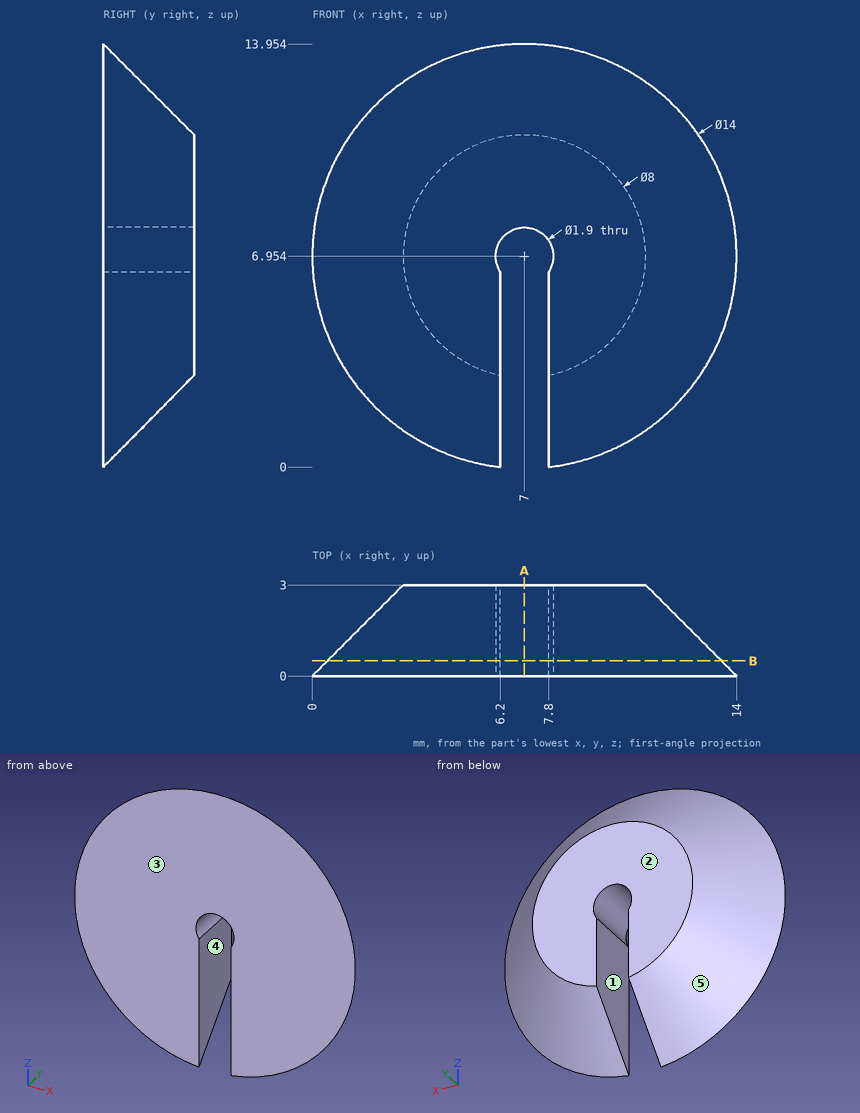
Source: three-view drawing plus pictorial views. Frame: mm from the lowest corner of the part. A direction names the side the tool comes from. Round coordinates to 2 decimals unless told otherwise and drop trailing zeros. Loops run counter-clockwise (first coordinate to the right, second up) from the corner with the lowest first, then second, coordinate; pieces in that order, holes last. Notation, with made-up numbers: M 72.5,14.25 L 111.5,14.25 A20 cw 111.5,36.25 Z; hole C 8,81 d9. An arc over 180 degrees is marked long. Put each result on its own line as item: value.
(1) First-contact query: pin 1 (1.5 mm diameter, centred on x = 3.5, y = 1, fed in from +Z); pin 2 (1.5 mm diameter, centred on x = 7, y = 2.5, fed in from +Z). Flat tips, straight axial feed; report the tip coordinate or a pass-through.
Solutions:
pin 1: z = 12.83
pin 2: z = 12.2
(2) Section A-A, the plane x = 7. Return loops of the section in (y, z).
Solutions:
outline: M 0,7.9 L 3,7.9 L 3,10.95 L 0,13.95 Z
(3) Section B-B, the plane y = 0.5. Return loops of the section in (x, z).
Solutions:
outline: M 6.2,0.5 L 6.2,6.44 A0.95 cw long 7.8,6.44 L 7.8,0.5 A6.5 ccw long Z
(4) Pull-direction query (X, two-part tool) for the marked faces 3, 4 and 5; classes: released by +X, released by -X, zero draft, split by the parting line, or undercut.
Solutions:
face 3: zero draft
face 4: undercut
face 5: split by the parting line
(5) Access query for the marked faces 1 and 2. Directions: +Z, -Z, +X, -X, +Y, -Y. A direction counts if a zero-diameter tool reaches every point of the face in a straight line with its end or side. Return the directions, or none.
Solutions:
face 1: -Z, +Y, -Y
face 2: +Z, -Z, +X, -X, +Y
(6) Ray query, line 1 (X direction, y = 0.6, z = 5.5); line 2 (Z direction, x = 3, y = 2.2); line 3 (X direction, y = 1.95, z = 4.5). Return the intervals inside material, ascending. Write a range as [from, to].
Solutions:
line 1: [0.77, 6.2], [7.8, 13.23]
line 2: [4.3, 9.61]
line 3: [2.59, 6.2], [7.8, 11.41]
